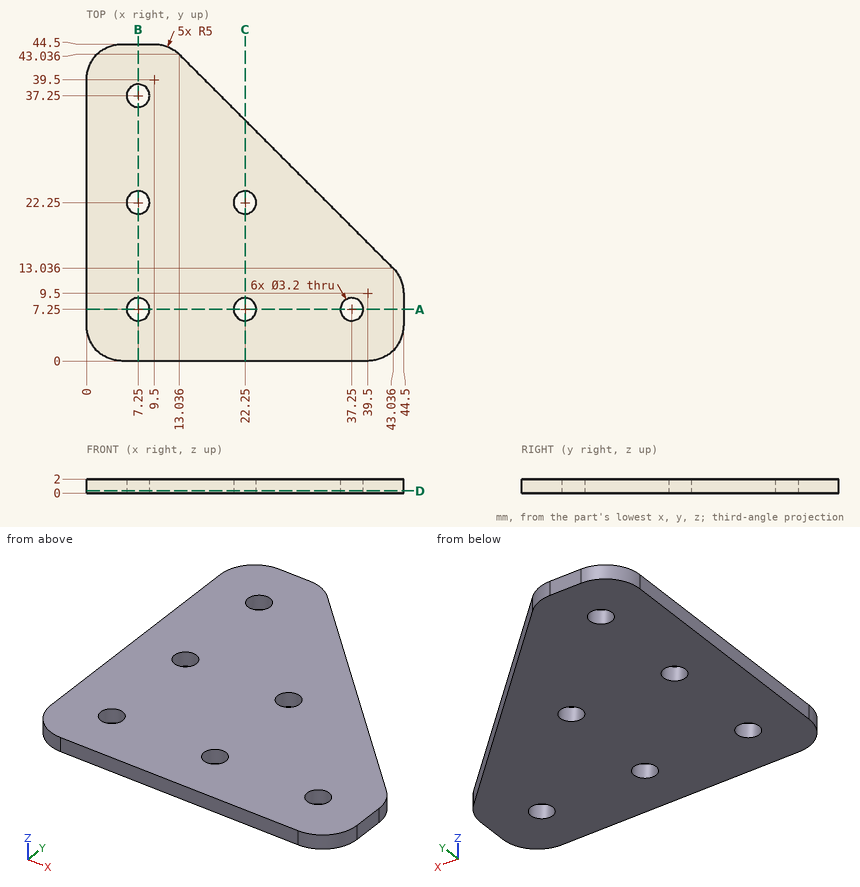
Design review of the part shown in the three views and the two pictorial views. Dimensions are in mm from the part's minimum x, y and z. Give positions to 0.01 mm unless a question says otherwise; leave off trailing zeros. Loops run counter-clockwise (first coordinate to the right, second up) from the corner with the lowest first, then second, coordinate; pieces in that order, holes last. Notation, with made-up numbers: (75, -8.75) -> (88, -8.75) arc R21 ccw to (88, 19.25) -> close; hole circle Ø11 at (79.5, -12). An arc over 180 degrees is marked (long way). Answer as a JSON object with one key per item and string values. Group by question number.
Q1. Insertion check: pin 1 (1 mm diameter, centred on y = 25.5, z = 1.5, fed in from +X); pin 2 (1 mm diameter, centred on x = 39.5, z = 1.5, fed in from +Y). Each pin has a flat end and moves straight along its axis. Give the tip position at first contact, or say it passes through.
Q2. Wall thickness on line 1 along Y through (x, z) = (7.25, 0.55); line 2 along X through (y, z) = (7, 1.7); line 3 along Y through (x, z) = (6, 1.2): over which ranges is each line inside the solid? List them lowest first.
Q3. Take a section at A-A (y = 7.25). Write out the cut boundary in (x, z).
Q4. Take a section at D-D (z = 0.35). State how many separate pieces and enclosed holes the cut face has, plus the area to 3 significant figures.
Q5. Take a section at C-C (x = 22.25). Write out the cut boundary in (y, z).
Answer below:
{
 "1": {"pin 1": "stops at x = 31.07", "pin 2": "stops at y = 17.07"},
 "2": {"line 1": "y = 0 to 5.65, 8.85 to 20.65, 23.85 to 35.65, 38.85 to 44.5", "line 2": "x = 0 to 5.67, 8.83 to 20.67, 23.83 to 35.67, 38.83 to 44.5", "line 3": "y = 0 to 6.25, 8.25 to 21.25, 23.25 to 36.25, 38.25 to 44.5"},
 "3": {"outline": "(0, 0) -> (5.65, 0) -> (5.65, 2) -> (0, 2) -> close; (8.85, 0) -> (20.65, 0) -> (20.65, 2) -> (8.85, 2) -> close; (23.85, 0) -> (35.65, 0) -> (35.65, 2) -> (23.85, 2) -> close; (38.85, 0) -> (44.5, 0) -> (44.5, 2) -> (38.85, 2) -> close"},
 "4": {"separate pieces": "1", "enclosed holes": "6", "area": "1,370 mm2"},
 "5": {"outline": "(0, 0) -> (5.65, 0) -> (5.65, 2) -> (0, 2) -> close; (8.85, 0) -> (20.65, 0) -> (20.65, 2) -> (8.85, 2) -> close; (23.85, 0) -> (33.82, 0) -> (33.82, 2) -> (23.85, 2) -> close"}
}
